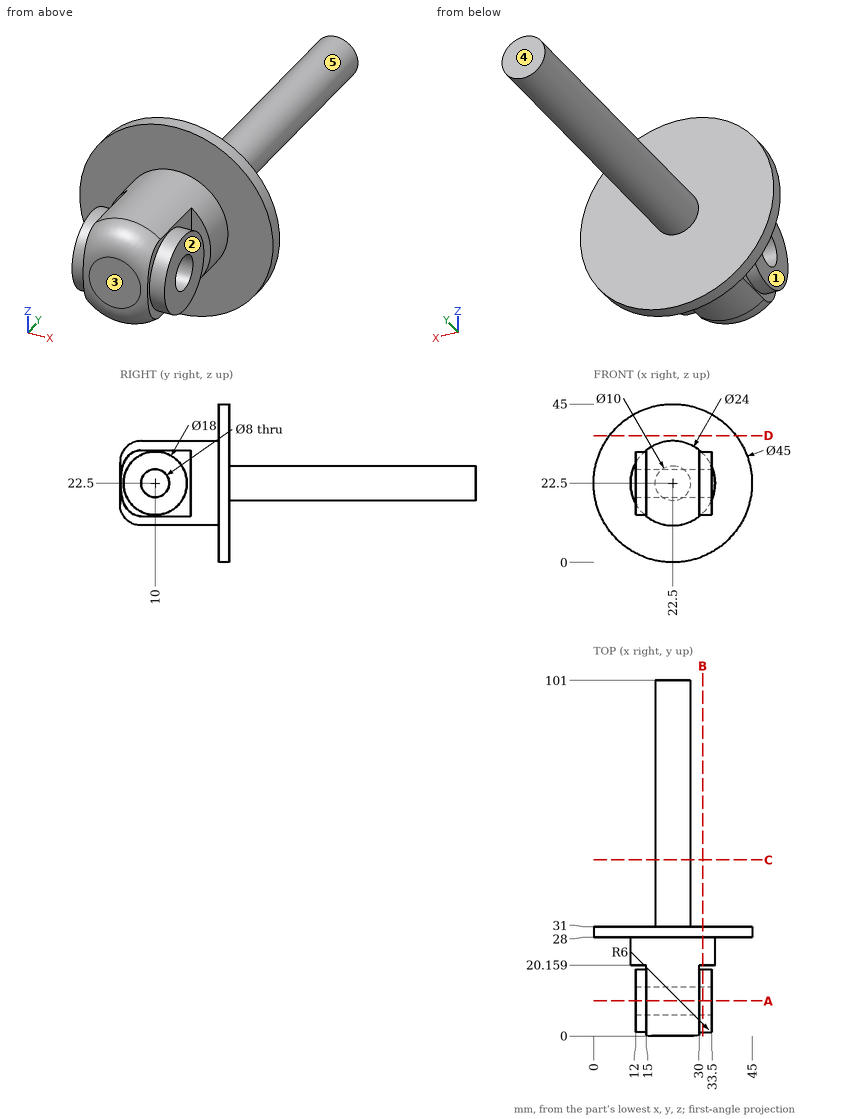
Job drawing, mm, ordinate dimensions from the low corner. One solid piece. A direction names the side the tool comes from. Give positions to 0.01 mm unless a question says otherwise; leave off trailing zeros. Order: outer loops, then holes, each group sorted by start corner. A loop starts at its lowest first (then second) coordinate and runs counter-clockwise, first axis right, second up. Notation, with made-up numbers: (-5.5, -4) -> (23.5, -4) arc R18 ccw to (23.5, 25) -> close; hole circle Ø8 at (17.25, 28). An arc over 180 degrees is marked (long way). Return JSON: item names as keys, results as strings.
Q1. Saw through at A-A (y = 10). Write the cut outline in (x, z).
Working result:
{"outline": "(12, 13.5) -> (15, 13.5) -> (15, 13.13) arc R12 ccw to (30, 13.13) -> (30, 13.5) -> (33.5, 13.5) -> (33.5, 18.5) -> (12, 18.5) -> close; (12, 26.5) -> (33.5, 26.5) -> (33.5, 31.5) -> (30, 31.5) -> (30, 31.87) arc R12 ccw to (15, 31.87) -> (15, 31.5) -> (12, 31.5) -> close"}
Q2. Drill centre lines: line 1 (Z direction, x = 22.5, y = 10); line 2 (Y direction, x = 23, z = 22.5); line 3 (Y direction, x = 37, z = 6.5). Where is each one in solid material? Low to high.
Working result:
{"line 1": "10.5 to 18.5, 26.5 to 34.5", "line 2": "0 to 6, 14 to 101", "line 3": "28 to 31"}
Q3. Saw through at B-B (x = 31). Write the cut outline in (y, z), then the cut area to 3 significant figures.
Working result:
{"outline": "circle Ø18 at (10, 22.5); (20.16, 14.03) -> (28, 14.03) -> (28, 1.67) -> (31, 1.67) -> (31, 43.33) -> (28, 43.33) -> (28, 30.97) -> (20.16, 30.97) -> close; hole circle Ø8 at (10, 22.5)", "area": "462 mm²"}
Q4. Saw through at D-D (z = 36). Write the cut outline in (x, y), then the cut area to 3 significant figures.
Working result:
{"outline": "(4.5, 28) -> (40.5, 28) -> (40.5, 31) -> (4.5, 31) -> close", "area": "108 mm²"}
Q5. Saw through at C-C (y = 50). Write the cut outline in (x, z), then the cut area to 3 significant figures.
Working result:
{"outline": "circle Ø10 at (22.5, 22.5)", "area": "78.5 mm²"}
Q6. Flat gauge pins, fed straight in: pin 1 (3 mm diameter, centred on x = 35.5, z = 39, fed in from -Y); pin 2 (15 mm diameter, centred on y = 15, z = 22, fed in from +X); pin 3 (1.5 mm diameter, centred on x = 27.5, y = 40, fed in from +Z). Where does each tip first touch, or does it go through?
Working result:
{"pin 1": "y = 28", "pin 2": "x = 34.5", "pin 3": "z = 25.13"}
Q7. Which spindle directions (+Z, -Z, +X, -X, +Y, -Y) get a long thin tool onto all of the face, cutting with end or side? Do the marked faces 1, 2, 3, 4 and 5. Say none if no direction does.
Working result:
{"face 1": "+Z, -Z, -X, -Y", "face 2": "+Z, -Z, +X, -Y", "face 3": "+Z, -Z, +X, -X, -Y", "face 4": "+Z, -Z, +X, -X, +Y", "face 5": "+Y"}
